Work out the finished part from the listing and answer in its coordinate system (mm). Face numbers are marked on the shaded views. A direction names the side the tool comes from. Coordinates: 2 decimals unless noted, no trailing zeros. Order: outer loops, then holes, each group sorted by start corner. A loop starts at its lowest first (then second) coordinate and runs counter-clockwise, first axis right, second up. Notation, with made-up numbers: M 57,63 L 83,63 A30 cw 83,98 Z; hole C -36.75,-22.5 d9. An arc over 180 degrees is marked long. Use a Markdown table: item, result.
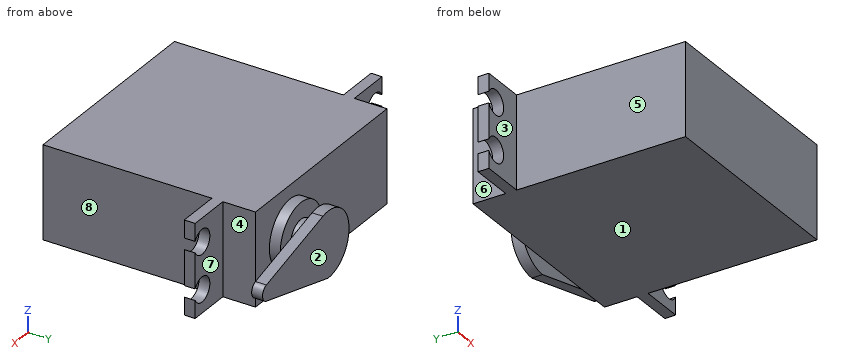
from build123d import *

# Parameters (mm, degrees)
SKETCH1_W           = 38
SKETCH1_H           = 17
BOSS_EXTRUDE1_DEPTH = 39
BOSS_EXTRUDE2_DEPTH = 2
SKETCH3_R           = 6
BOSS_EXTRUDE3_DEPTH = 2
SKETCH4_R           = 3
BOSS_EXTRUDE4_DEPTH = 3
BOSS_EXTRUDE5_DEPTH = 2


with BuildPart() as part:
    # Sketch1 → Boss-Extrude1 (new body)
    with BuildSketch(Plane(origin=(0, 0, 0), x_dir=(1, 0, 0), z_dir=(0, 1, 0))):
        Rectangle(SKETCH1_W, SKETCH1_H)
    extrude(amount=BOSS_EXTRUDE1_DEPTH)

    # Sketch2 → Boss-Extrude2 (add)
    with BuildSketch(Plane(origin=(0, 31, 0), x_dir=(1, 0, 0), z_dir=(0, 1, 0))):
        with BuildLine():
            Line((19, 8.5), (27, 8.5))
            Line((27, 8.5), (27, 5.280776406))
            ThreePointArc((27, 5.280776406), (22.75, 4.25), (27, 3.219223594))
            Line((27, 3.219223594), (27, -3.219223594))
            ThreePointArc((27, -3.219223594), (22.75, -4.25), (27, -5.280776406))
            Line((27, -5.280776406), (27, -8.5))
            Line((27, -8.5), (19, -8.5))
            Line((19, -8.5), (19, 8.5))
        make_face()
    boss_extrude2 = extrude(amount=BOSS_EXTRUDE2_DEPTH)

    # Mirror1: Boss-Extrude2 across plane
    add(boss_extrude2.mirror(Plane(origin=(0, 0, 0), x_dir=(0, 0, 1), z_dir=(1, 0, 0))))

    # Sketch3 → Boss-Extrude3 (add)
    with BuildSketch(Plane(origin=(0, 39, 0), x_dir=(1, 0, 0), z_dir=(0, 1, 0))):
        with Locations((9, 0)):
            Circle(SKETCH3_R)
    extrude(amount=BOSS_EXTRUDE3_DEPTH)

    # Sketch4 → Boss-Extrude4 (add)
    with BuildSketch(Plane(origin=(0, 41, 0), x_dir=(1, 0, 0), z_dir=(0, 1, 0))):
        with Locations((9, 0)):
            Circle(SKETCH4_R)
    extrude(amount=BOSS_EXTRUDE4_DEPTH)

    # Sketch5 → Boss-Extrude5 (add)
    with BuildSketch(Plane(origin=(0, 44, 0), x_dir=(1, 0, 0), z_dir=(0, 1, 0))):
        with BuildLine():
            Line((9, 6), (26.869837254, 1.453691991))
            ThreePointArc((26.869837254, 1.453691991), (27.99997757, 0.008202936), (26.885714286, -1.449560102))
            Line((26.885714286, -1.449560102), (10.542857143, -5.798240409))
            ThreePointArc((10.542857143, -5.798240409), (3.050653714, -0.777996641), (9, 6))
        make_face()
    extrude(amount=BOSS_EXTRUDE5_DEPTH)


solid = part.part
1. For a pull along Y with two mould halves and no side action, classify the marked faces 1, 2, 3 and 4 as +Y half, -Y half, draft (parallel to the pull), parting line (faces both ways), or undercut.
Answers below:
| item | result |
|---|---|
| face 1 | draft |
| face 2 | +Y half |
| face 3 | -Y half |
| face 4 | undercut |
2. For the marked faces 5, 6, 7 and 8, determine the directions among +Z, -Z, +X, -X, +Y, -Y from which every point of the face is accessible in a straight line to the end or side of a thin tool.
Answers below:
| item | result |
|---|---|
| face 5 | +Z, -Z, -X, -Y |
| face 6 | +Z, -Z, -X, +Y |
| face 7 | +Z, -Z, +X |
| face 8 | +Z, -Z, +X, -Y |
3. Section B-B on z = -4.25 is taken. Determine the outline of the cut face in (x, y), then the cut area to 3 significant figures.
Answers below:
| item | result |
|---|---|
| outline | M -22.75,31 L -19,31 L -19,0 L 19,0 L 19,31 L 22.75,31 L 22.75,33 L 19,33 L 19,39 L 13.24,39 L 13.24,41 L 4.76,41 L 4.76,39 L -19,39 L -19,33 L -22.75,33 Z; M 4.76,44 L 15.88,44 L 15.88,46 L 4.76,46 Z |
| area | 1,540 mm² |
4. Section C-C on z = 0 is taken. Determine the outline of the cut face in (x, y), then the cut area to 3 significant figures.
Answers below:
| item | result |
|---|---|
| outline | M -27,31 L -19,31 L -19,0 L 19,0 L 19,31 L 27,31 L 27,33 L 19,33 L 19,39 L 15,39 L 15,41 L 12,41 L 12,44 L 28,44 L 28,46 L 3,46 L 3,44 L 6,44 L 6,41 L 3,41 L 3,39 L -19,39 L -19,33 L -27,33 Z |
| area | 1,610 mm² |
5. Flat-ended cylindrical pins translate along their axes: P1, Ø5, axis at y = 20, z = 0.5, coming from the +X side; P2, Ø4, axis at x = -22, z = 1, coming from the -Y side; P3, Ø1, axis at x = -4, y = 40.5, coming from the +Z side; P4, Ø6.5, axis at y = 37, z = -1.5, coming from the -X side. Find the tip coordinate at first contact, or state that the pin passes through.
Answers below:
| item | result |
|---|---|
| P1 | x = 19 |
| P2 | y = 31 |
| P3 | through |
| P4 | x = -19 |
6. Section D-D on x = 25 is taken. Determine the outline of the cut face in (y, z).
Answers below:
| item | result |
|---|---|
| outline | M 31,-8.5 L 33,-8.5 L 33,-6.5 L 31,-6.5 Z; M 31,-2 L 33,-2 L 33,2 L 31,2 Z; M 31,6.5 L 33,6.5 L 33,8.5 L 31,8.5 Z; M 44,-1.93 L 46,-1.93 L 46,1.95 L 44,1.95 Z |
7. Section A-A on x = -25 is taken. Determine the outline of the cut face in (y, z), then the cut area to 3 significant figures.
Answers below:
| item | result |
|---|---|
| outline | M 31,-8.5 L 33,-8.5 L 33,-6.5 L 31,-6.5 Z; M 31,-2 L 33,-2 L 33,2 L 31,2 Z; M 31,6.5 L 33,6.5 L 33,8.5 L 31,8.5 Z |
| area | 16.0 mm² |
8. Find the intervals of material crossed by probe 1 along Z at (x, y) = (-25, 32.25); probe 2 along Y at (x, z) = (4.5, 1); probe 3 along X at (y, z) = (31.9, 4.25), in increasing order.
Answers below:
| item | result |
|---|---|
| probe 1 | -8.5 to -6.5, -2 to 2, 6.5 to 8.5 |
| probe 2 | 0 to 41, 44 to 46 |
| probe 3 | -22.75 to 22.75 |
